from build123d import *

# Parameters (mm, degrees)
F1_DEPTH    = 0.4
F2_DEPTH    = 6.35
F4_DEPTH    = 7.9375
F6_DEPTH    = 6.35
F7_T1_DEPTH = 14.2875


# Not quite as in the source:
# - a fillet or chamfer that OpenCascade refuses, or shapes differently, is made with other operations: its cross-section is extruded or revolved along the edge and cut away or added
# - a pattern or mirror of a feature is missing from the dataset's text; its kind, count and spacing are read off the source's solid


with BuildPart() as f1:
    # F0 (on Front) → F1 (new body)
    with BuildSketch(Plane.XZ):
        with BuildLine():
            ThreePointArc((-12.7, 15.01775), (-11.0611032579, 14.3388967421), (-10.38225, 12.7))
            ThreePointArc((-10.38225, 12.7), (-12.7, 10.38225), (-15.01775, 12.7))
            Line((-15.01775, 12.7), (-15.01775, -12.7000000336))
            ThreePointArc((-15.01775, -12.7000000336), (-12.7000000168, -10.38225), (-10.38225, -12.7))
            ThreePointArc((-10.38225, -12.7), (-11.0611032579, -14.3388967421), (-12.7, -15.01775))
            Line((-12.7, -15.01775), (12.7, -15.01775))
            ThreePointArc((12.7, -15.01775), (11.0611032579, -11.0611032579), (15.01775, -12.7))
            Line((15.01775, -12.7), (15.01775, 12.7))
            ThreePointArc((15.01775, 12.7), (11.0611032579, 11.0611032579), (12.7, 15.01775))
            Line((12.7, 15.01775), (-12.7, 15.01775))
        make_face()
        with BuildLine():
            ThreePointArc((-10.38225, -12.7), (-12.7000000168, -10.38225), (-15.01775, -12.7000000336))
            ThreePointArc((-15.01775, -12.7000000336), (-14.3388967302, -14.338896754), (-12.7, -15.01775))
            ThreePointArc((-12.7, -15.01775), (-11.0611032579, -14.3388967421), (-10.38225, -12.7))
        make_face()
        with BuildLine():
            ThreePointArc((-15.01775, 12.7), (-12.7, 10.38225), (-10.38225, 12.7))
            ThreePointArc((-10.38225, 12.7), (-11.0611032579, 14.3388967421), (-12.7, 15.01775))
            ThreePointArc((-12.7, 15.01775), (-14.3388967421, 14.3388967421), (-15.01775, 12.7))
        make_face()
        with BuildLine():
            ThreePointArc((15.01775, 12.7), (14.3388967421, 14.3388967421), (12.7, 15.01775))
            ThreePointArc((12.7, 15.01775), (11.0611032579, 11.0611032579), (15.01775, 12.7))
        make_face()
        with BuildLine():
            ThreePointArc((12.7, -15.01775), (14.3388967421, -14.3388967421), (15.01775, -12.7))
            ThreePointArc((15.01775, -12.7), (11.0611032579, -11.0611032579), (12.7, -15.01775))
        make_face()
        with BuildLine():
            ThreePointArc((-15.01775, 12.7), (-14.3388967421, 14.3388967421), (-12.7, 15.01775))
            Line((-12.7, 15.01775), (-15.01775, 15.01775))
            Line((-15.01775, 15.01775), (-15.01775, 12.7))
        make_face()
        with BuildLine():
            Line((15.01775, 15.01775), (12.7, 15.01775))
            ThreePointArc((12.7, 15.01775), (14.3388967421, 14.3388967421), (15.01775, 12.7))
            Line((15.01775, 12.7), (15.01775, 15.01775))
        make_face()
        with BuildLine():
            Line((15.01775, -15.01775), (15.01775, -12.7))
            ThreePointArc((15.01775, -12.7), (14.3388967421, -14.3388967421), (12.7, -15.01775))
            Line((12.7, -15.01775), (15.01775, -15.01775))
        make_face()
        with BuildLine():
            ThreePointArc((-12.7, -15.01775), (-14.3388967302, -14.338896754), (-15.01775, -12.7000000336))
            Line((-15.01775, -12.7000000336), (-15.01775, -15.01775))
            Line((-15.01775, -15.01775), (-12.7, -15.01775))
        make_face()
    extrude(amount=F1_DEPTH)

    # F0 (on Front) → F2 (join)
    with BuildSketch(Plane.XZ):
        with BuildLine():
            ThreePointArc((-15.01775, 12.7), (-12.7, 10.38225), (-10.38225, 12.7))
            ThreePointArc((-10.38225, 12.7), (-11.0611032579, 14.3388967421), (-12.7, 15.01775))
            ThreePointArc((-12.7, 15.01775), (-14.3388967421, 14.3388967421), (-15.01775, 12.7))
        make_face()
        with BuildLine():
            ThreePointArc((-10.38225, -12.7), (-12.7000000168, -10.38225), (-15.01775, -12.7000000336))
            ThreePointArc((-15.01775, -12.7000000336), (-14.3388967302, -14.338896754), (-12.7, -15.01775))
            ThreePointArc((-12.7, -15.01775), (-11.0611032579, -14.3388967421), (-10.38225, -12.7))
        make_face()
        with BuildLine():
            ThreePointArc((12.7, -15.01775), (14.3388967421, -14.3388967421), (15.01775, -12.7))
            ThreePointArc((15.01775, -12.7), (11.0611032579, -11.0611032579), (12.7, -15.01775))
        make_face()
    extrude(amount=-F2_DEPTH)

    # F0 (on Front) → F4 (join)
    with BuildSketch(Plane.XZ):
        with BuildLine():
            ThreePointArc((-15.01775, 12.7), (-12.7, 10.38225), (-10.38225, 12.7))
            ThreePointArc((-10.38225, 12.7), (-11.0611032579, 14.3388967421), (-12.7, 15.01775))
            ThreePointArc((-12.7, 15.01775), (-14.3388967421, 14.3388967421), (-15.01775, 12.7))
        make_face()
        with BuildLine():
            ThreePointArc((15.01775, 12.7), (14.3388967421, 14.3388967421), (12.7, 15.01775))
            ThreePointArc((12.7, 15.01775), (11.0611032579, 11.0611032579), (15.01775, 12.7))
        make_face()
    extrude(amount=-F4_DEPTH)

    # F5 (on plane+point) → F6 (join)
    with BuildSketch(Plane.XY.offset(12.7)):
        with BuildLine():
            Line((15.01775, 5.61975), (15.01775, 7.9375))
            Line((15.01775, 7.9375), (10.38225, 7.9375))
            Line((10.38225, 7.9375), (10.38225, 5.61975))
            ThreePointArc((10.38225, 5.61975), (12.7, 3.302), (15.01775, 5.61975))
        make_face()
    f6 = extrude(amount=F6_DEPTH)

    # F6_copies: F6 across plane
    add(f6.mirror(Plane(origin=(0, 0, 0), x_dir=(0, 0, -1), z_dir=(-1, 0, 0))))

    # F7: fillet of radius 1.5875 on 4 edges, made by hand

    # F7_s2 → F7_t1 (cut)
    with BuildSketch(Plane.XY.offset(8.73125)):
        with BuildLine():
            ThreePointArc((15.01775, 6.35), (14.5527820151, 7.4725320151), (13.43025, 7.9375))
            Line((13.43025, 7.9375), (15.01775, 7.9375))
            Line((15.01775, 7.9375), (15.01775, 6.35))
        make_face()
        with BuildLine():
            ThreePointArc((11.96975, 7.9375), (10.8472179849, 7.4725320151), (10.38225, 6.35))
            Line((10.38225, 6.35), (10.38225, 7.9375))
            Line((10.38225, 7.9375), (11.96975, 7.9375))
        make_face()
        with BuildLine():
            ThreePointArc((-10.38225, 6.35), (-10.8472179849, 7.4725320151), (-11.96975, 7.9375))
            Line((-11.96975, 7.9375), (-10.38225, 7.9375))
            Line((-10.38225, 7.9375), (-10.38225, 6.35))
        make_face()
        with BuildLine():
            ThreePointArc((-13.43025, 7.9375), (-14.5527820151, 7.4725320151), (-15.01775, 6.35))
            Line((-15.01775, 6.35), (-15.01775, 7.9375))
            Line((-15.01775, 7.9375), (-13.43025, 7.9375))
        make_face()
    extrude(amount=F7_T1_DEPTH, mode=Mode.SUBTRACT)


solid = f1.part
Can you work these out from the model? Positions are in its coordinate system, mm. A direction names the side the tool comes from. Coordinates: 2 decimals unless noted, no trailing zeros. Write each loop counter-clockwise with the first axis right and the second up, starting at its lowest first coordinate (ties: lowest second). Pieces come first, ordered by that corner, then holes. Notation, with made-up numbers: (52, -2) -> (95, -2) arc R27 cw to (95, 31) -> close; hole circle Ø7 at (-40, -27.75). An arc over 180 degrees is marked (long way). Write item = value, one per line.
(1) On a 3-axis mill with a long thin cutter (end or side, diameter ignored), from which of +Z, -Z, +X, -X, +Y, -Y can I reach the whole of each face in a straight line? I mean faces 4 (the face through (13, 6.35, -13)), 5 (the face through (-14.6, 0, -14.5)), 6 (the face through (14.5, 0, 14.6)), 7 (the face through (-10.835, 7.46, 14.715)). Say none if no direction works.
Verdict:
face_4 = -Z, +X, -X, +Y
face_5 = -Z, -X, +Y
face_6 = +Z, +X
face_7 = +Z, -Z, +Y
(2) Imagine slicing it at C-C (y = 7). Please give me the cut outline in (x, z), and give its area (3 significant figures).
Verdict:
outline = (-14.88, 11.91) arc R2.32 ccw to (-10.52, 11.91) -> (-10.52, 19.05) -> (-14.88, 19.05) -> close; (10.52, 11.91) arc R2.32 ccw to (14.88, 11.91) -> (14.88, 19.05) -> (10.52, 19.05) -> close
area = 71.9 mm^2
(3) Thinking about a two-plate mould opening in Y: for faces 1 (the face through (-12.802, 3.031, 10.384)), 2 (the face through (14.5, 0, -14.5)), 3 (the face through (13, 6, 19.05)), which applies, +Y half, -Y half, draft (parallel to the pull), parting line (faces both ways), or undercut?
Verdict:
face_1 = undercut
face_2 = +Y half
face_3 = draft
(4) If I drill on probe 1 along X at (y, z) = (0.5, -12.5); probe 2 along Y at (x, z) = (14.5, -2); probe 3 along Z at (x, y) = (12, 0.5), over which ranges is the centre line in solid material (lowest first)?
Verdict:
probe_1 = -15.01 to -10.39, 10.39 to 15.01
probe_2 = -0.4 to 0
probe_3 = -14.91 to -10.49, 10.49 to 14.91
(5) Imagine slicing it at A-A (y = 0.75). Please give me the cut outline in (x, z), and give its area (3 significant figures).
Verdict:
outline = circle Ø4.64 at (-12.7, -12.7); circle Ø4.64 at (-12.7, 12.7); circle Ø4.64 at (12.7, -12.7); circle Ø4.64 at (12.7, 12.7)
area = 67.5 mm^2
(6) For pin 1 (1 mm diameter, centred on x = 9, y = 1.5, fed in from -Z); pin 2 (0.7 mm diameter, centred on x = 14, z = -13.5, fed in from +Y), each with a flat end and sliding along its axis, tell me the tip position at first contact or that it passes through.
Verdict:
pin_1 = through
pin_2 = 6.35
